Autodesk Inventor part; units mm, degrees
ref_plane "Start Plane" through (0, 0, -3.7262) normal (0, 0, 1) x (1, 0, 0)
ref_plane "End Plane" through (0, 0, 356.7124) normal (0, 0, 1) x (1, 0, 0)
ref_plane "Work Plane4" through (0, -10, -3.7262) normal (0, 0.3492, -0.9371) x (1, 0, 0)
ref_plane "Start Plane" through (0, 0, -3.7262) normal (0, 0, 1) x (1, 0, 0)
ref_plane "End Plane" through (0, 0, 356.7124) normal (0, 0, 1) x (1, 0, 0)
sketch "Sketch" plane through (0, 0, 0) normal (0, 0, 1) x (1, 0, 0)
  line L0 (-10, -7) -> (-10, 7)
  line L1 (-7, 10) -> (7, 10)
  line L2 (10, 7) -> (10, -7)
  line L3 (7, -10) -> (-7, -10)
  arc A0 (-10, -7) -> (-7, -10) centre (-7, -7) ccw
  arc A1 (-7, 10) -> (-10, 7) centre (-7, 7) ccw
  arc A2 (10, 7) -> (7, 10) centre (7, 7) ccw
  arc A3 (7, -10) -> (10, -7) centre (7, -7) ccw
  arc A4 (-7, 8) -> (-8, 7) centre (-7, 7) ccw
  line L4 (-7, 8) -> (7, 8)
  arc A5 (8, 7) -> (7, 8) centre (7, 7) ccw
  line L5 (8, 7) -> (8, -7)
  arc A6 (7, -8) -> (8, -7) centre (7, -7) ccw
  line L6 (7, -8) -> (-7, -8)
  arc A7 (-8, -7) -> (-7, -8) centre (-7, -7) ccw
  line L7 (-8, -7) -> (-8, 7)
  line L8 (0, 14.8698) -> (0, -14.8698) construction
  line L9 (-14.8698, 0) -> (14.8698, 0) construction
  dimension "d7" = 3
  dimension "d10" = 20
  dimension "d11" = 20
  dimension "d12" = 2
  dimension "d15" = 10
  dimension "d16" = 10
extrude "Body" add sketch "Sketch" along normal up to surface (360.4385 mm away) from surface at -3.7262
sketch "Sketch3" plane through (0, 0, 0) normal (0, 0, 1) x (1, 0, 0)
  line L0 (0, 0) -> (10, 0)
ref_plane "Work Plane3" through (0, 0, 0) normal (0, -1, 0) x (1, 0, 0)
sketch "Sketch4" plane through (0, 0, 0) normal (0, -1, 0) x (1, 0, 0)
  line L0 (-2, -3.7262) -> (12, -3.7262)
  line L1 (-2, 356.7124) -> (12, 356.7124)
  dimension "d18" = 360.4385
ref_plane "Work Plane4" through (0, -10, -3.7262) normal (0, 0.3492, -0.9371) x (1, 0, 0)
split "Split1" plane through (0, -10, -3.7262) removes the side toward (0, 0.3492, -0.9371)
ref_plane "Work Plane6" through (-10, 0, 356.7124) normal (0.7897, 0, 0.6134) x (0.6134, 0, -0.7897)
split "Split3" plane through (-10, 0, 356.7124) removes the side toward (0.7897, 0, 0.6134)
ref_plane "Work Plane7" through (310, 12.1423, 345.0892) normal (0, 0.7562, 0.6544) x (1, 0, 0)
split "Split4" plane through (310, 12.1423, 345.0892) removes the side toward (0, 0.7562, 0.6544)
ref_plane "Work Plane8" through (310, -1.2506, 355.9809) normal (0, -0.6544, 0.7562) x (1, 0, 0)
split "Split5" plane through (310, -1.2506, 355.9809) removes the side toward (0, -0.6544, 0.7562)
equation "\"d7\" = G_IR"
equation "\"d10\" = G_H"
equation "\"d11\" = G_W"
equation "\"d12\" = G_T"
equation "\"d15\" = 0.5 * d10"
equation "\"d16\" = 0.5 * d11"
equation "\"d3\" = G_L"
equation "\"G_W\" = 20"
equation "\"G_H\" = 20"
equation "\"G_T\" = 2"
equation "\"G_IR\" = 3"
equation "\"G_L\" = d18"
equation "\"G_OFFSET_START\" = 3.72616"
equation "\"G_OFFSET_END\" = 12.87375"
equation "\"d13\" = -G_OFFSET_START"
equation "\"d14\" = G_OFFSET_END + B_L"
equation "\"B_L\" = 343.83862"
properties part number "ISO 12633-2 - 20x20x2 - 360,44" material "Steel, Mild"
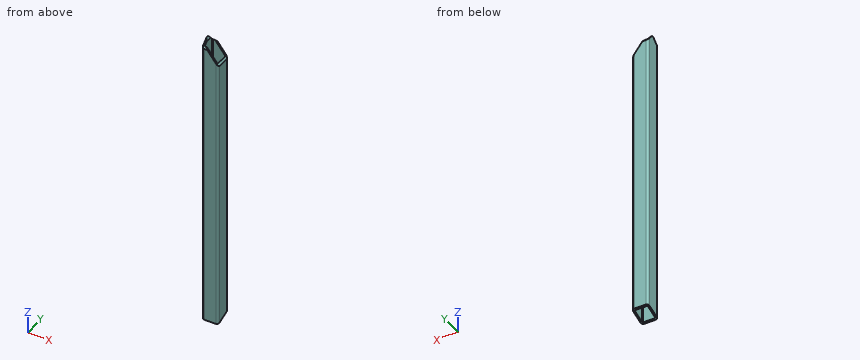
For this review, take the finished solid that the model builds, in its own axes (mm). Give positions to 0.01 mm unless a question says otherwise; leave off trailing zeros. Loops run counter-clockwise (first coordinate to the right, second up) from the corner with the lowest first, then second, coordinate; pieces in that order, holes last. Notation, with made-up numbers: M 39.5,14 L 69.5,14 A29 cw 69.5,52 Z; hole C 58.25,83 d3. An arc over 180 degrees is marked long. Put each result on its own line as item: value. Start each with the question number.
(1) Add section B-B, the plane x = 2. Write out the cut boundary in (y, z).
(2) Add section A-A, the plane z = 161.5. Write out the cut boundary in (x, y).
(3) Wall thickness on L1, parallel to Y at x = 3.5, z = 105; L2, parallel to X at y = -6.5, z = 338: over which ranges is each line inside the solid? List them lowest first.
(4) For pin 1 (4 mm diameter, centred on x = -5.5, y = -4.5, fed in from +Z), flat-tipped, find the tip position at first contact; note if it passes through.
Result:
1. outline: M -10,-3.73 L -8,-2.98 L -8,341.26 L -10,341.26 Z; M 8,2.98 L 10,3.73 L 10,341.26 L 8,341.26 Z
2. outline: M -10,-7 A3 ccw -7,-10 L 7,-10 A3 ccw 10,-7 L 10,7 A3 ccw 7,10 L -7,10 A3 ccw -10,7 Z; hole M -8,-7 A1 ccw -7,-8 L 7,-8 A1 ccw 8,-7 L 8,7 A1 ccw 7,8 L -7,8 A1 ccw -8,7 Z
3. L1: y = -10 to -8, 8 to 10
3. L2: x = -10 to -8
4. pin 1: passes through
